```python
from build123d import *

# Parameters (mm, degrees)
SKETCH2_R          = 8.255
CUT_EXTRUDE1_DEPTH = 11.43
CIRPATTERN1_COUNT  = 3
SKETCH3_R          = 4.826
CUT_EXTRUDE2_DEPTH = 12.7


with BuildPart() as part:
    # Sketch1 → Revolve1 (revolve)
    with BuildSketch(Plane.XY):
        with BuildLine():
            Line((0, 19.05), (0, 0))
            Line((0, 0), (-38.1, 0))
            add(Edge.make_bspline(
                [(0, 19.05), (-25.41, 19.05), (-38.1, 6.316666667), (-38.1, 0)],
                knots=[0, 0, 0, 0, 1, 1, 1, 1], degree=3))
        make_face()
    revolve(axis=Axis((0, 0, 0), (-1, 0, 0)))

    # Sketch2 → Cut-Extrude1 (cut)
    with BuildSketch(Plane(origin=(0, 19.05, 0), x_dir=(1, 0, 0), z_dir=(0, 1, 0))):
        with Locations((-12.7, 0)):
            Circle(SKETCH2_R)
    cut_extrude1 = extrude(amount=-CUT_EXTRUDE1_DEPTH, mode=Mode.SUBTRACT)

    # CirPattern1: Cut-Extrude1 ×3 about axis
    cirpattern1_axis = Axis((0, 0, 0), (1, 0, 0))
    for i in range(1, CIRPATTERN1_COUNT):
        add(cut_extrude1.rotate(cirpattern1_axis, i * 360 / CIRPATTERN1_COUNT), mode=Mode.SUBTRACT)

    # Sketch3 → Cut-Extrude2 (cut)
    with BuildSketch(Plane(origin=(0, 0, 0), x_dir=(0, 0, -1), z_dir=(1, 0, 0))):
        Circle(SKETCH3_R)
    extrude(amount=-CUT_EXTRUDE2_DEPTH, mode=Mode.SUBTRACT)


solid = part.part
```
Geometry: final body of the model. Coordinates: model frame, mm. A direction names the side the tool comes from. Coordinates: 2 decimals unless noted, no trailing zeros. Answer in a Markdown table with one row per item. Add a question column.
Q1. Line query: L1, parallel to Z at x = -12.7, y = 15 (3 decimals); L2, parallel to X at y = -8, z = 10; L3, parallel to Y at x = -7, z = 5. Output: solid intervals per line, ascending.
Q2. Mould query, pull axis X, two halves, no side actions, for faces 1 (the cylindrical face through (-4.826, 12.092, -2.48)), 2 (the cylindrical face through (-4.826, -8.193, -9.232)), 3 (the cylindrical face through (-6.261, -2.937, 3.83)), 4 (the flat face through (-12.7, 0, 0)). Classes: released by +X, released by -X, zero draft, split by the parting line, or undercut.
Q3. Reachability of faces 5 (the flat face through (-13, 7.62, 0)), 6 (the flat face through (0, 4, 4)), 7 (the flat face through (-12.82, -3.91, -6.54)) from +Z, -Z, +X, -X, +Y, -Y: full face, straight path, thin tool, end or side. Return the list, or none.
Q4. Contact query for flat-ended pins moving along their axis: P1, Ø18, axis at x = -14, z = 3, coming from the +Y side; P2, Ø5, axis at y = -2.5, z = 0, coming from the +X side; P3, Ø3, axis at x = -14.5, y = 2.5, coming from the -Z side; P4, Ø6, axis at y = 0, z = -6.5, coming from the -X side. Output: stop coordinate, or through.
Completed:
| question | item | result |
|---|---|---|
| 1 | L1 | z = -9.736 to -8.255, 8.255 to 9.736 |
| 1 | L2 | x = -27.04 to -20.73, -4.67 to 0 |
| 1 | L3 | y = -18.03 to -9.78, -6.58 to 7.62 |
| 2 | face 1 | undercut |
| 2 | face 2 | undercut |
| 2 | face 3 | zero draft |
| 2 | face 4 | released by +X |
| 3 | face 5 | +Y |
| 3 | face 6 | +Z, -Z, +X, +Y, -Y |
| 3 | face 7 | none |
| 4 | P1 | stops at y = 18.64 |
| 4 | P2 | stops at x = 0 |
| 4 | P3 | stops at z = -17.7 |
| 4 | P4 | stops at x = -37.1 |
